For this review, use the dimensioned drawing (mm, ordinates from the lowest corner) and the shaded views. Coordinates: 2 decimals unless noted, no trailing zeros. Loops run counter-clockwise (first coordinate to the right, second up) from the corner with the lowest first, then second, coordinate; pieces in that order, holes last. Notation, with made-up numbers: M 73.5,-26.5 L 94.5,-26.5 A17 ccw 94.5,5.5 Z; hole C 23.5,46.5 d10. An arc over 180 degrees is marked long. Write item = value, one per line. Start each with the question number.
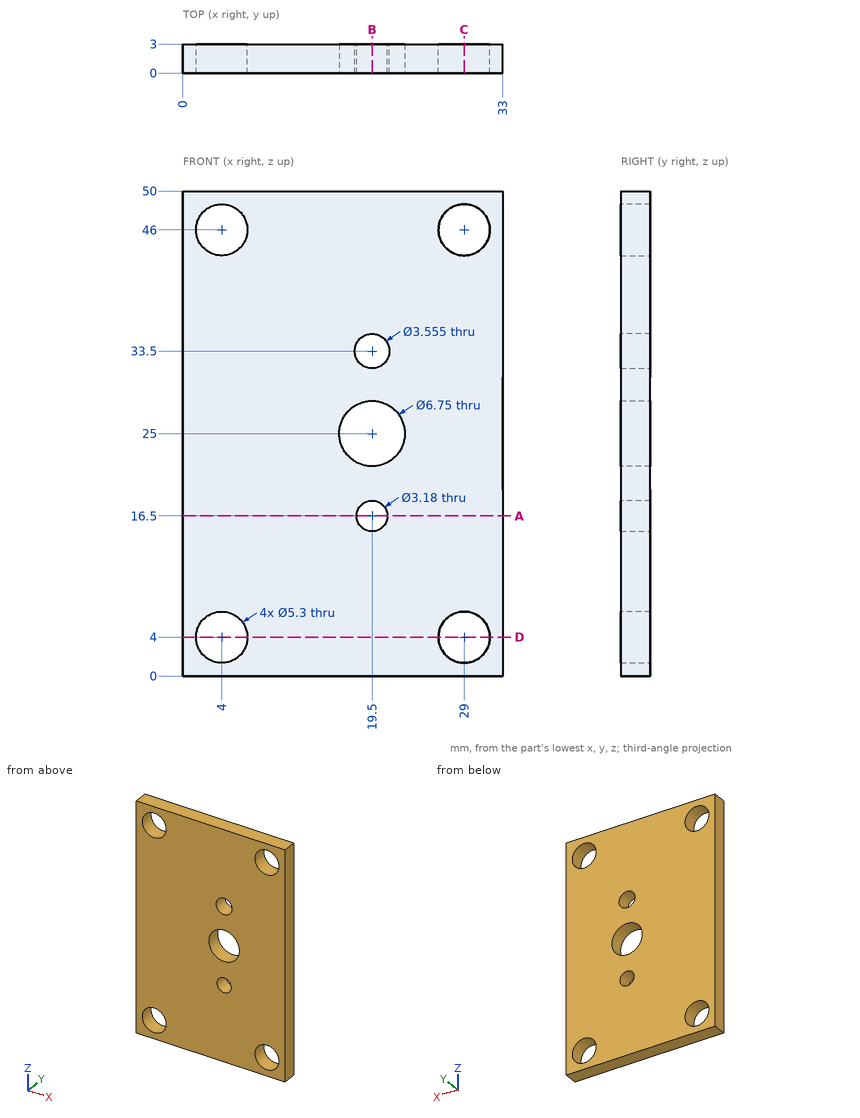
Q1. Add section D-D on z = 4. State the section outline as (x, y) points.
Q2. Add section B-B on x = 19.5. State the section outline as (y, z) points (1 decimal).
Q3. Add section A-A on z = 16.5. State the section outline as (x, y) points.
Q4. Clearance check with a flat-ended pin moving along its axis: P1, Ø3, axis at x = 19.5, z = 33.5, coming from the +Y side. State where the tip first meets the part, or that it passes through.
Q5. To check wall thickness, follow line 1 (X direction, y = 1.95, z = 46); line 2 (Z direction, x = 27, y = 1.05); line 3 (Z direction, x = 3.5, y = 1.2). State the ranges of each line that lie inside material, in increasing order. Write a range as from..to.
Q6. Add section C-C on x = 29. State the section outline as (y, z) points, plus the area to 3 significant figures.
Values follow:
q1.outline = M 0,0 L 1.35,0 L 1.35,3 L 0,3 Z; M 6.65,0 L 26.35,0 L 26.35,3 L 6.65,3 Z; M 31.65,0 L 33,0 L 33,3 L 31.65,3 Z
q2.outline = M 0,0 L 3,0 L 3,14.9 L 0,14.9 Z; M 0,18.1 L 3,18.1 L 3,21.6 L 0,21.6 Z; M 0,28.4 L 3,28.4 L 3,31.7 L 0,31.7 Z; M 0,35.3 L 3,35.3 L 3,50 L 0,50 Z
q3.outline = M 0,0 L 17.91,0 L 17.91,3 L 0,3 Z; M 21.09,0 L 33,0 L 33,3 L 21.09,3 Z
q4.P1 = through
q5.line_1 = 0..1.35, 6.65..26.35, 31.65..33
q5.line_2 = 0..2.26, 5.74..44.26, 47.74..50
q5.line_3 = 0..1.4, 6.6..43.4, 48.6..50
q6.outline = M 0,0 L 3,0 L 3,1.35 L 0,1.35 Z; M 0,6.65 L 3,6.65 L 3,43.35 L 0,43.35 Z; M 0,48.65 L 3,48.65 L 3,50 L 0,50 Z
q6.area = 118 mm2
